Model file for the job. Use its own axes, mm. A direction names the side the tool comes from. Give positions to 0.01 mm unless a question says otherwise; leave off trailing zeros. Order: outer loops, then holes, each group sorted by start corner. A loop starts at its lowest first (then second) coordinate and runs counter-clockwise, first axis right, second up. Notation, with made-up numbers: (48, 29.5) -> (107, 29.5) arc R18 cw to (107, 44.5) -> close; hole circle Ø2 at (-16, 25). An arc over 180 degrees is marked (long way). Use CSV: the item, a comma, the result in double quotes. Start each with the question number.
1. Cut at D-D on y = 5.5. List the corners of the cut face in (x, z), then the cut area to 3 significant figures.
2. Drop flat-ended pins along their axis: pin 1 (1.5 mm diameter, centred on x = 5, y = 8, fed in from -Z); pin 2 (1 mm diameter, centred on x = -4, y = -7, fed in from +Z). Give the stop position or say it passes through.
3. 3-axis set-ups, long thin cutter, end or side, ignore diameter. For faces 1 (the flat face through (5, -5, 1)), 2 (the cylindrical face through (-1.4, 10.66, 0.49)): which of +Z, -Z, +X, -X, +Y, -Y reach the whole face in a straight line?
4. Cut at A-A on y = 0. List the corners of the cut face in (x, z).
5. Cut at C-C on z = 5.5. List the corners of the cut face in (x, y), then the cut area to 3 significant figures.
6. Wall check: line 1 (Z direction, x = 8.75, y = -5.75); line 2 (Z direction, x = -4.75, y = 2.5); line 3 (X direction, y = -2.5, z = 3.75). Give the ranges that are in metal, low to high. Write a range as from..to.
```python
from build123d import *

# Parameters (mm, degrees)
F0_R     = 10.75
F0_R_2   = 6.5
F0_R_3   = 4
F1_DEPTH = 1
F2_DEPTH = 3.5
F3_DEPTH = 6.5


with BuildPart() as f1:
    # F0 (on Top) → F1 (new body)
    with BuildSketch(Plane.XY):
        Circle(F0_R)
        Circle(F0_R_2, mode=Mode.SUBTRACT)
        Circle(F0_R_2)
        Circle(F0_R_3, mode=Mode.SUBTRACT)
        Circle(F0_R_3)
    extrude(amount=F1_DEPTH)

    # F0 (on Top) → F2 (join)
    with BuildSketch(Plane.XY):
        Circle(F0_R_2)
        Circle(F0_R_3, mode=Mode.SUBTRACT)
        Circle(F0_R_3)
    extrude(amount=F2_DEPTH)

    # F0 (on Top) → F3 (join)
    with BuildSketch(Plane.XY):
        Circle(F0_R_3)
    extrude(amount=F3_DEPTH)


solid = f1.part
```
Verdict:
1,outline,"(-9.24, 0) -> (9.24, 0) -> (9.24, 1) -> (3.46, 1) -> (3.46, 3.5) -> (-3.46, 3.5) -> (-3.46, 1) -> (-9.24, 1) -> close"
1,area,"35.8 mm^2"
2,pin 1,"z = 0"
2,pin 2,"z = 1"
3,face 1,"+Z"
3,face 2,"+Z, -Z"
4,outline,"(-10.75, 0) -> (10.75, 0) -> (10.75, 1) -> (6.5, 1) -> (6.5, 3.5) -> (4, 3.5) -> (4, 6.5) -> (-4, 6.5) -> (-4, 3.5) -> (-6.5, 3.5) -> (-6.5, 1) -> (-10.75, 1) -> close"
5,outline,"circle Ø8 at (0, 0)"
5,area,"50.3 mm^2"
6,line 1,"0..1"
6,line 2,"0..3.5"
6,line 3,"-3.12..3.12"
